The listing builds one solid part. Answer for the finished solid, in the listing's coordinates (mm). A direction names the side the tool comes from. Coordinates: 2 decimals unless noted, no trailing zeros. Order: outer loops, then holes, each group sorted by start corner. A loop starts at its lowest first (then second) coordinate and runs counter-clockwise, first axis right, second up. Notation, with made-up numbers: (70.5, 53.25) - (85.5, 53.25) arc R26 cw to (85.5, 71.25) - close; hole circle Ø5 at (42.5, 68). An arc over 180 degrees is marked (long way). Use one line per item in the form item = value. Start each with the question number.
Item 1: Consider line 1 along Y through (x, z) = (0, 11); line 2 along Z through (x, y) = (-10.5, 13); line 3 along Z through (x, y) = (-4, -22.5). Determine where each line is inside the solid, lowest interval first. Write a range as [from, to].
Item 2: Section B-B, the plane x = -9 is taken. Write down the section's boundary in (y, z), and give its area (3 significant figures).
Item 3: The mould has two halves that part along Y. Classify faces 1 (the flat face through (19, -19.05, 13)), 2 (the flat face through (25, 0, 19.05)), 3 (the cylindrical face through (-2.75, -12.4, 9.66)), 4 (the cylindrical face through (69.85, 0.19, 12.61)): released by +Y, released by -Y, zero draft, split by the parting line, or undercut.
Item 4: Section A-A, the plane y = 0 is taken. Write down the section's boundary in (x, z).
Item 5: Section D-D, the plane x = 33.5 is taken. Write down the section's boundary in (y, z), and give its area (3 significant figures).
Item 6: Each of these flat-tipped pins is pushed along its axis until it touches: pin 1 Ø10 at (x, z) = (10.5, 15.5) entering from -Y; pin 2 Ø2 at (y, z) = (3, 8.5) entering from +X; pin 3 Ø14 at (x, z) = (58, 13.5) entering from -Y. Where does it stop, or does it pass through?
Item 7: Section C-C, the plane z = 17 is taken. Write down the section's boundary in (x, y).
Item 8: A tool of negligible diameter and unlimited length cuts with its end or side. For faces 5 (the flat face through (38.1, 16, 13)), 6 (the flat face through (38.1, -16, 13)), 7 (the flat face through (19, 19.05, 13)), from which of +Z, -Z, +X, -X, +Y, -Y can it reach the whole face along a straight path? Write none if from no direction.
Autodesk Inventor part; units mm, degrees
ref_plane "YZ Plane" through (0, 0, 0) normal (1, 0, 0) x (0, 1, 0)
ref_plane "XZ Plane" through (0, 0, 0) normal (0, 1, 0) x (-1, 0, 0)
ref_plane "XY Plane" through (0, 0, 0) normal (0, 0, 1) x (1, 0, 0)
sketch "Sketch1" plane through (0, 0, 0) normal (0, 0, 1) x (1, 0, 0)
  arc A0 (0, 25.4) -> (0, -25.4) centre (0, 0) ccw
  arc A1 (50.8, -25.4) -> (50.8, 25.4) centre (50.8, 0) ccw
  line L0 (0, 25.4) -> (50.8, 25.4)
  line L1 (0, -25.4) -> (50.8, -25.4)
  dimension "d2" = 50.8
  dimension "d3" = 50.8
  dimension "d4" = 50.8
extrude "Extrusion1" add sketch "Sketch1" along normal blind 6.35
sketch "Sketch2" plane through (0, 0, 6.35) normal (0, 0, 1) x (1, 0, 0)
  arc A0 (0, 25.4) -> (0, -25.4) centre (0, 0) ccw
  line L0 (0, -25.4) -> (50.8, -25.4)
  arc A1 (50.8, -25.4) -> (50.8, 25.4) centre (50.8, 0) ccw
  line L1 (50.8, 25.4) -> (0, 25.4)
  arc A2 (0, 19.05) -> (0, -19.05) centre (0, 0) ccw
  arc A3 (64.999, -12.7) -> (64.999, 12.7) centre (50.8, 0) ccw
  line L2 (0, -19.05) -> (38.1, -19.05)
  line L3 (0, 19.05) -> (38.1, 19.05)
  line L4 (64.999, -12.7) -> (38.1, -12.7)
  line L5 (64.999, 12.7) -> (38.1, 12.7)
  circle A4 centre (0, 0) radius 12.7
  line L6 (38.1, 19.05) -> (38.1, 12.7)
  line L7 (38.1, -12.7) -> (38.1, -19.05)
  dimension "d8" = 38.1
  dimension "d9" = 38.1
  dimension "d10" = 38.1
  dimension "d11" = 38.1
  dimension "d16" = 25.4
  dimension "d17" = 25.4
extrude "Extrusion2" add sketch "Sketch2" along normal blind 12.7 contours L3 L6 L5 A3 L4 L7 L2 A2
sketch "Sketch3" plane through (0, 0, 6.35) normal (0, 0, 1) x (1, 0, 0)
  circle A0 centre (0, 0) radius 12.7
  dimension "d20" = 25.4
extrude "Extrusion3" cut sketch "Sketch3" against normal through all
sketch "Sketch4" plane through (0, 0, 19.05) normal (0, 0, 1) x (1, 0, 0)
  circle A0 centre (0, 0) radius 12.7
  arc A1 (0, 19.05) -> (0, -19.05) centre (0, 0) ccw
  line L0 (0, -19.05) -> (38.1, -19.05)
  line L1 (38.1, -19.05) -> (38.1, -12.7)
  line L2 (38.1, -12.7) -> (64.999, -12.7)
  arc A2 (64.999, -12.7) -> (64.999, 12.7) centre (50.8, 0) ccw
  line L3 (64.999, 12.7) -> (38.1, 12.7)
  line L4 (38.1, 12.7) -> (38.1, 19.05)
  line L5 (38.1, 19.05) -> (0, 19.05)
  circle A3 centre (50.8, 0) radius 6.35
  dimension "d23" = 12.7
extrude "Extrusion4" add sketch "Sketch4" along normal blind 6.35 contours A3
properties part number "HW 6 Part 6"
Response:
q1.line_1 = [-19.05, -12.7], [12.7, 19.05]
q1.line_2 = [0, 19.05]
q1.line_3 = [0, 6.35]
q2.outline = (-23.75, 0) - (-8.96, 0) - (-8.96, 19.05) - (-16.79, 19.05) - (-16.79, 6.35) - (-23.75, 6.35) - close; (8.96, 0) - (23.75, 0) - (23.75, 6.35) - (16.79, 6.35) - (16.79, 19.05) - (8.96, 19.05) - close
q2.area = 387 mm2
q3.face_1 = released by -Y
q3.face_2 = zero draft
q3.face_3 = undercut
q3.face_4 = split by the parting line
q4.outline = (-25.4, 0) - (-12.7, 0) - (-12.7, 19.05) - (-19.05, 19.05) - (-19.05, 6.35) - (-25.4, 6.35) - close; (12.7, 0) - (76.2, 0) - (76.2, 6.35) - (69.85, 6.35) - (69.85, 19.05) - (57.15, 19.05) - (57.15, 25.4) - (44.45, 25.4) - (44.45, 19.05) - (12.7, 19.05) - close
q5.outline = (-25.4, 0) - (25.4, 0) - (25.4, 6.35) - (19.05, 6.35) - (19.05, 19.05) - (-19.05, 19.05) - (-19.05, 6.35) - (-25.4, 6.35) - close
q5.area = 806 mm2
q6.pin_1 = -19.05
q6.pin_2 = 69.74
q6.pin_3 = -12.7
q7.outline = (0, -19.05) - (38.1, -19.05) - (38.1, -12.7) - (65, -12.7) arc R19.05 ccw to (65, 12.7) - (38.1, 12.7) - (38.1, 19.05) - (0, 19.05) arc R19.05 ccw to start; hole circle Ø25.4 at (0, 0)
q8.face_5 = +Z, +X, +Y
q8.face_6 = +Z, +X, -Y
q8.face_7 = +Z, +X, -X, +Y
